CAD build for the part. Positions are in the model's coordinates, mm. Face numbers are marked on the shaded views. A direction names the side the tool comes from. Coordinates: 2 decimals unless noted, no trailing zeros. Loops run counter-clockwise (first coordinate to the right, second up) from the corner with the lowest first, then second, coordinate; pieces in that order, holes last. Notation, with made-up numbers: (-6, 20) -> (28, 20) arc R33 ccw to (28, 54) -> close; hole circle Ø11 at (69, 24). An arc over 180 degrees is marked (long way). Return JSON: item names as keys, results as strings. Group by question number.
(1) Saw through at D-D on z = -8. Write the cut outline in (x, y).
(2) Mould opens along Y. For the marked faces 1, 2 and 3 say: pulls with the +Y half, pulls with the -Y half, needs draft (parallel to the pull), parting line crosses it, or undercut.
(3) Saw through at C-C on x = -42. Write the cut outline in (y, z).
(4) Saw through at B-B on y = -37. Write the cut outline in (x, z).
(5) Flat gauge pins, fed straight in: pin 1 Ø4.5 at (x, y) = (-16.5, -4) entering from +Z; pin 2 Ø14.5 at (x, y) = (11.12, -34.47) entering from +Z; pin 3 Ø24 at (y, z) = (-26, 44) entering from +X. Where does each tip first touch, or does it go through?
(6) Saw through at A-A on z = 41.5. Write the cut outline in (x, y).
(7) Tool access for the marked faces 4, 5 and 6: list every direction of +Z, -Z, +X, -X, +Y, -Y with a clear straight run to the whole face (end or side of a thin tool).
(8) Probe L1, parallel to X at y = -4, z = 28.5; L2, parallel to X at y = -3.5, z = 44.45; L3, parallel to Y at x = 23, z = 12.5. List the from-to ranges inside material, lowest first.
```python
from build123d import *

# Parameters (mm, degrees)
F0_W     = 63.5
F0_H     = 60.198
F1_DEPTH = 9.398
F3_DEPTH = 12.7
F5_DEPTH = 9.398


with BuildPart() as f1:
    # F0 (on Front) → F1 (new body)
    with BuildSketch(Plane.XZ):
        with Locations((-31.75, 30.099)):
            Rectangle(F0_W, F0_H)
        with BuildLine():
            ThreePointArc((-55.2396252751, 44.1290847957), (-46.5901332262, 52.387728278), (-39.4916252751, 42.7632755798))
            Line((-39.4916252751, 42.7632755798), (-39.4916252751, 25.4))
            ThreePointArc((-39.4916252751, 25.4), (-46.5009541347, 17.4653953282), (-55.2396252751, 23.442373583))
            Line((-55.2396252751, 23.442373583), (-55.2396252751, 44.1290847957))
        make_face(mode=Mode.SUBTRACT)
        with BuildLine():
            ThreePointArc((-33.3522260189, 43.7816642225), (-27.1048819761, 52.4199260723), (-17.6042260189, 47.5839761388))
            Line((-17.6042260189, 47.5839761388), (-17.6042260189, 25.4))
            ThreePointArc((-17.6042260189, 25.4), (-26.3222239844, 17.4888395764), (-33.3522260189, 26.9317744576))
            Line((-33.3522260189, 26.9317744576), (-33.3522260189, 43.7816642225))
        make_face(mode=Mode.SUBTRACT)
        Polygon((47.498, 0), (0, 60.198), (0, 0), align=None)
    extrude(amount=F1_DEPTH)

    # F2 (on Top) → F3 (join)
    with BuildSketch(Plane.XY):
        Polygon((47.5135771375, 0), (-63.4844228625, 0), (-64.0543534469, -16.2460061286), (-9.3824228625, -57.658), (47.5135771375, -57.658), align=None)
        with BuildLine():
            ThreePointArc((17.4686820134, -34.4697237222), (4.7694330104, -34.5673817862), (17.4656782032, -34.2744306938))
            ThreePointArc((17.4656782032, -34.2744306938), (17.4679310165, -34.3720656582), (17.4686820134, -34.4697237222))
        make_face(mode=Mode.SUBTRACT)
        with BuildLine():
            ThreePointArc((26.8592325641, -33.9853970117), (33.1085706899, -27.4408549802), (39.5562287539, -33.7901039832))
            ThreePointArc((39.5562287539, -33.7901039832), (33.3038868178, -40.1393529863), (26.8592325641, -33.9853970117))
        make_face(mode=Mode.SUBTRACT)
    extrude(amount=-F3_DEPTH)

    # F4 (on Right) → F5 (join)
    with BuildSketch(Plane.YZ):
        Polygon((-9.7489070876, 0), (-9.7489070876, 60.2996), (-57.3169094876, 0), align=None)
    extrude(amount=-F5_DEPTH)


solid = f1.part
```
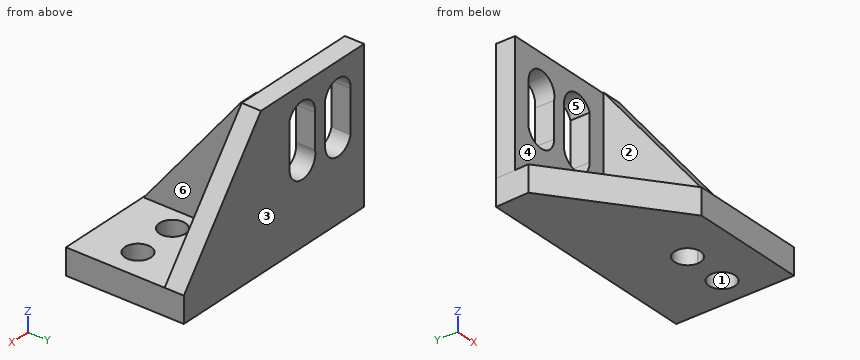
Geometry results:
{
 "1": {"outline": "(-64.05, -16.25) -> (-9.38, -57.66) -> (47.51, -57.66) -> (47.51, 0) -> (-63.48, 0) -> close; hole circle Ø12.7 at (11.12, -34.47); hole circle Ø12.7 at (33.21, -33.79)"},
 "2": {"face 1": "undercut", "face 2": "needs draft", "face 3": "pulls with the +Y half"},
 "3": {"outline": "(-32.95, -12.7) -> (0, -12.7) -> (0, 19.58) -> (-9.4, 19.58) -> (-9.4, 0) -> (-32.95, 0) -> close; (-9.4, 50.42) -> (0, 50.42) -> (0, 60.2) -> (-9.4, 60.2) -> close"},
 "4": {"outline": "(-36.66, -12.7) -> (5.29, -12.7) -> (5.29, 0) -> (0, 0) -> (0, 25.75) -> (-9.4, 25.75) -> (-9.4, 0) -> (-36.66, 0) -> close; (16.94, -12.7) -> (27.73, -12.7) -> (27.73, 0) -> (16.94, 0) -> close; (38.69, -12.7) -> (47.51, -12.7) -> (47.51, 0) -> (38.69, 0) -> close"},
 "5": {"pin 1": "z = 60.2", "pin 2": "z = 0", "pin 3": "x = 0"},
 "6": {"outline": "(-63.5, -9.4) -> (-55.24, -9.4) -> (-55.24, 0) -> (-63.5, 0) -> close; (-39.49, -9.4) -> (-33.35, -9.4) -> (-33.35, 0) -> (-39.49, 0) -> close; (-17.6, -9.4) -> (14.75, -9.4) -> (14.75, 0) -> (-17.6, 0) -> close; (-9.4, -24.58) -> (0, -24.58) -> (0, -9.75) -> (-9.4, -9.75) -> close"},
 "7": {"face 4": "+Z, +X, -X", "face 5": "+Y, -Y", "face 6": "+Z, +X, -Y"},
 "8": {"L1": "-63.5 to -55.24, -39.49 to -33.35, -17.6 to 25.01", "L2": "-63.5 to -55.25, -39.31 to -33.38, -17.6 to 12.43", "L3": "-9.4 to 0"}
}
